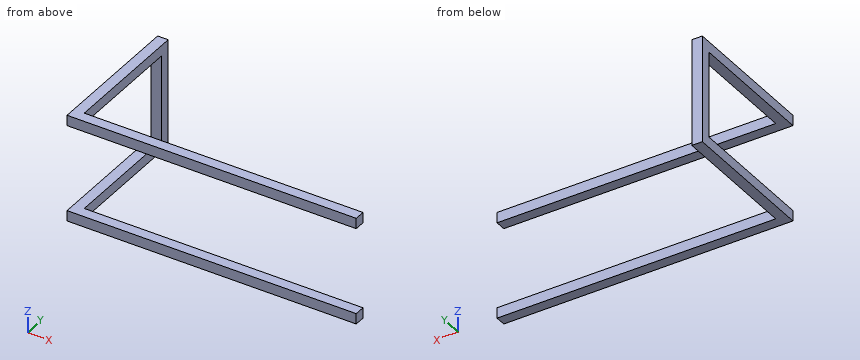
from build123d import *

# Parameters (mm, degrees)
EXTRUDE_1_DEPTH = 40
SKETCH_6_W      = 40
SKETCH_6_H      = 408.4
EXTRUDE_2_DEPTH = 40


with BuildPart() as part:
    # Sketch 2 → Extrude 1 (new body)
    with BuildSketch(Plane.XY.offset(164.2)):
        Polygon((-475, 0), (585, 0), (585, -40), (-515, -40), (-515, 500), (-475, 500), (-475, 460), align=None)
    extrude(amount=EXTRUDE_1_DEPTH)


with BuildPart() as body_2:
    # Mirror 4: mirrored copy
    add(part.part.mirror(Plane.XY))


with BuildPart() as part_1:
    add(part.part)

    add(body_2.part)  # Extrude 2 merges body 2
    # Sketch 6 → Extrude 2 (add)
    with BuildSketch(Plane(origin=(0, 500, 0), x_dir=(1, 0, 0), z_dir=(0, 1, 0))):
        with Locations((-495, 0)):
            Rectangle(SKETCH_6_W, SKETCH_6_H)
    extrude(amount=-EXTRUDE_2_DEPTH)


solid = part_1.part
Check sheet for the modelled part. Datum: model origin and axes. Units: mm. Round coordinates to 2 decimals unless told otherwise and drop trailing zeros. Order: outer loops, then holes, each group sorted by start corner. A loop starts at its lowest first (then second) coordinate and runs counter-clockwise, first axis right, second up.
Q1. Scan lines: L1, parallel to X at y = 448, z = -165.5; L2, parallel to Y at x = -425.5, z = -173. Record each from-to range of solid material in increasing order.
Filled sheet:
L1: x = -515 to -475
L2: y = -40 to 0
Q2. Cross-section at D-D, the plane z = 73.5. Enter the section's corners in (x, y), plus the area to 3 significant figures.
Filled sheet:
outline: (-515, 460) - (-475, 460) - (-475, 500) - (-515, 500) - close
area: 1,600 mm2
Q3. Cross-section at B-B, the plane x = 209. Enter the section's corners in (y, z), plus the area to 3 significant figures.
Filled sheet:
outline: (-40, -204.2) - (0, -204.2) - (0, -164.2) - (-40, -164.2) - close; (-40, 164.2) - (0, 164.2) - (0, 204.2) - (-40, 204.2) - close
area: 3,200 mm2
Q4. Cross-section at A-A, the plane y = 295.5. Enter the section's corners in (x, z), plus the area to 3 significant figures.
Filled sheet:
outline: (-515, -204.2) - (-475, -204.2) - (-475, -164.2) - (-515, -164.2) - close; (-515, 164.2) - (-475, 164.2) - (-475, 204.2) - (-515, 204.2) - close
area: 3,200 mm2
Q5. Cross-section at C-C, the plane z = 178. Enter the section's corners in (x, y).
Filled sheet:
outline: (-515, -40) - (585, -40) - (585, 0) - (-475, 0) - (-475, 500) - (-515, 500) - close
Q6. Depth check by flat-ended pin: P1, Ø12, axis at x = -203.5, z = -185, coming from the +Y side; P2, Ø12, axis at x = -488.5, z = -15.5, coming from the -Y side. Enter the tip coordinate at first touch or a pass-through.
Filled sheet:
P1: stops at y = 0
P2: stops at y = 460
